Could you check a few things on this model? Use its own coordinates, in mm. A direction names the side the tool comes from. Coordinates: 2 decimals unless noted, no trailing zeros. Order: outer loops, then holes, each group sorted by start corner. A loop starts at its lowest first (then second) coordinate and runs counter-clockwise, first axis right, second up. Notation, with made-up numbers: (87.5, -29.5) -> (114.5, -29.5) arc R27 cw to (114.5, 0.5) -> close; hole circle Ø9 at (61.5, 42.25). An arc over 180 degrees is marked (long way). Put each result on its own line as item: value. Start each with the question number.
Q1. If we section it at A-A (x = 0): Please give me the cut outline in (y, z) (3 decimals), and give its area (3 significant figures).
Q2. If we section it at C-C (z = 48.5): Please give me the cut outline in (x, y), and give its area (3 significant figures).
Q3. For faces 4 (the face through (12.7, -6, 106)), 5 (the face through (-1.2, -6.3, 206.3)), which set-ups out of +Z, -Z, +X, -X, +Y, -Y let a thin tool reach every point of the face, with its end or its side?
Q4. We'd pull the mould along X, two halves only. Please class faces 1 (the face through (0, -12.7, 84)), 2 (the face through (-12.7, -6, 108)), 3 (the face through (-15.12, -6.26, -11.59)): +X half, -X half, draft (parallel to the pull), parting line (faces both ways), or undercut.
Q5. Will these pins go through, and if not, where does the flat tip stop? pin 1 (3 mm diameter, centred on x = -8.5, y = -3, fed in from -Z); pin 2 (1 mm diameter, centred on y = -7, z = 129.5, fed in from -X); pin 3 (4.5 mm diameter, centred on y = -5, z = 142.5, fed in from +X); pin 4 (12 mm diameter, centred on x = -3.5, z = 175.5, fed in from +Y).
Q6. Please list where these lines run through material, in increasing order: line 1 along Z through (x, y) = (8.5, -3.5); line 2 along X through (y, z) = (-1.25, 201); line 3 along Z through (x, y) = (-11.5, -6.5).
Q7. If we section it at B-B (y = -6.75): Count the separate pieces of the cut face and the enclosed holes in it, and give its area (3 significant figures).
from build123d import *

# Parameters (mm, degrees)
F0_R     = 19.05
F0_R_2   = 9.525
F1_DEPTH = 12.7
F2_R     = 1.6002


with BuildPart() as f1:
    # F0 (on Front) → F1 (new body)
    with BuildSketch(Plane.XZ):
        with BuildLine():
            Line((-12.7, 187.325), (-12.7, 25.597668))
            ThreePointArc((-12.7, 25.597668), (0, -28.575), (12.7, 25.597668))
            Line((12.7, 25.597668), (12.7, 187.325))
            ThreePointArc((12.7, 187.325), (0, 212.725), (-12.7, 187.325))
        make_face()
        Circle(F0_R, mode=Mode.SUBTRACT)
        with Locations((0, 196.85)):
            Circle(F0_R_2, mode=Mode.SUBTRACT)
    extrude(amount=F1_DEPTH)

    # F2
    f2_edges = [f1.edges().sort_by_distance(p)[0] for p in [
        (0, -12.7, 212.725),
        (12.7, -12.7, 106.461334),
        (0, -12.7, -28.575),
        (-12.7, -12.7, 106.461334),
        (12.7, 0, 106.461334),
        (0, 0, 212.725),
        (-12.7, 0, 106.461334),
        (0, 0, -28.575),
        (12.7, -6.35, 25.597668),
        (12.7, -6.35, 187.325),
        (-12.7, -6.35, 187.325),
        (-12.7, -6.35, 25.597668),
    ]]
    fillet(f2_edges, radius=F2_R)


solid = f1.part
The answers:
1. outline: (-12.7, -26.975) arc R1.6 ccw to (-11.1, -28.575) -> (-1.6, -28.575) arc R1.6 ccw to (0, -26.975) -> (0, -19.05) -> (-12.7, -19.05) -> close; (-12.7, 19.05) -> (0, 19.05) -> (0, 187.325) -> (-12.7, 187.325) -> close; (-12.7, 206.375) -> (0, 206.375) -> (0, 211.125) arc R1.6 ccw to (-1.6, 212.725) -> (-11.1, 212.725) arc R1.6 ccw to (-12.7, 211.125) -> close
1. area: 2,340 mm^2
2. outline: (-12.7, -11.1) arc R1.6 ccw to (-11.1, -12.7) -> (11.1, -12.7) arc R1.6 ccw to (12.7, -11.1) -> (12.7, -1.6) arc R1.6 ccw to (11.1, 0) -> (-11.1, 0) arc R1.6 ccw to (-12.7, -1.6) -> close
2. area: 320 mm^2
3. face 4: +X, +Y, -Y
3. face 5: +Y, -Y
4. face 1: draft
4. face 2: -X half
4. face 3: undercut
5. pin 1: z = -27.7
5. pin 2: x = -12.7
5. pin 3: x = 12.7
5. pin 4: y = 0
6. line 1: -27.28 to -17.05, 17.05 to 192.55, 201.15 to 210.26
6. line 2: -15.28 to -8.57, 8.57 to 15.28
6. line 3: -26.16 to -15.19, 15.19 to 207.79
7. separate pieces: 1
7. enclosed holes: 2
7. area: 5,880 mm^2
